```python
from build123d import *

# Parameters (mm, degrees)
F1_DEPTH = 25
F2_R     = 21.75
F3_DEPTH = 25.001
F4_SIZE  = 2


with BuildPart() as f1:
    # F0 (on Top) → F1 (new body)
    with BuildSketch(Plane.XY):
        Polygon((20, 34.641016), (-20, 34.641016), (-40, 0), (-20, -34.641016), (20, -34.641016), (40, 0), align=None)
    extrude(amount=F1_DEPTH)

    # F2 (on face) → F3 (cut, through all)
    with BuildSketch(Plane.XY.offset(25)):
        Circle(F2_R)
    extrude(amount=-F3_DEPTH, mode=Mode.SUBTRACT)

    # F4
    f4_edges = [f1.edges().sort_by_distance(p)[0] for p in [
        (-21.75, 0, 0),
        (-21.75, 0, 25),
    ]]
    chamfer(f4_edges, length=F4_SIZE)

    # F5 (on Front) → F6 (revolve, cut)
    with BuildSketch(Plane.XZ):
        Polygon((42.406738, 25.509455), (33.521101, 25.509455), (42.406738, 21.53198), align=None)
        Polygon((42.136625, 3.734692), (33.521101, -0.952422), (42.136625, -0.952422), align=None)
    revolve(axis=Axis((0, 0, 7.913062), (0, 0, -1)), mode=Mode.SUBTRACT)


solid = f1.part
```
Could you check a few things on this model? Use its own coordinates, in mm. Round coordinates to 2 decimals unless told otherwise and drop trailing zeros. Order: outer loops, then holes, each group sorted by start corner. A loop starts at its lowest first (then second) coordinate and runs counter-clockwise, first axis right, second up. Notation, with made-up numbers: (55.5, -14.75) -> (89.5, -14.75) arc R17 ccw to (89.5, -6.75) -> close; hole circle Ø10 at (59, 23.25). An arc over 180 degrees is marked (long way). One line per question, with ' | ' between items.
Q1. If we section it at B-B on x = 0: Write out the boundary of the cut face in (y, z).
Computed values:
outline: (-34.64, 0) -> (-23.75, 0) -> (-21.75, 2) -> (-21.75, 23) -> (-23.75, 25) -> (-34.64, 25) -> close; (21.75, 2) -> (23.75, 0) -> (34.64, 0) -> (34.64, 25) -> (23.75, 25) -> (21.75, 23) -> close
Q2. If I drill on line 1 (Y direction, x = 0, z = 10.5); line 2 (X direction, y = 1, z = 6.5); line 3 (X direction, y = -2.5, z = 19.5), over which ranges is the centre line in solid material (lowest first)? Write a range as from..to.
Computed values:
line 1: -34.64..-21.75, 21.75..34.64 | line 2: -39.42..-21.73, 21.73..39.42 | line 3: -38.56..-21.61, 21.61..38.56
Q3. If we section it at A-A on z = 6.5: Write out the boundary of the cut face in (x, y), plus the area to 3 significant figures.
Computed values:
outline: (-40, 0) -> (-20, -34.64) -> (20, -34.64) -> (40, 0) -> (20, 34.64) -> (-20, 34.64) -> close; hole circle Ø43.5 at (0, 0) | area: 2,670 mm²
Q4. I'm going to push flat-ended pins straight in: pin 1 (6 mm diameter, centred on x = -26, z = 5, fed in from +Y); pin 2 (6 mm diameter, centred on y = -8.5, z = 12, fed in from -X); pin 3 (2 mm diameter, centred on x = 31.5, z = 3.5, fed in from +Y). Where does each tip first touch, or does it pass through?
Computed values:
pin 1: y = 29.44 | pin 2: x = -36.82 | pin 3: y = 16.45
Q5. We'd pull the mould along X, two halves only. Please class faces 1 (the face through (-2.831, 21.565, 12.647)), 2 (the face through (18.424, -31.569, 0.697)), 3 (the face through (-24, 0, 0)), 4 (the face through (-36.552, -0.171, 0.697)): released by +X, released by -X, zero draft, split by the parting line, or undercut.
Computed values:
face 1: undercut | face 2: released by +X | face 3: zero draft | face 4: released by -X
